Input: dimensioned drawing with shaded views. Units: mm. Origin: part minimum x, y, z. A direction names the side the tool comes from. Coordinates: 2 decimals unless noted, no trailing zeros. Order: outer loops, then holes, each group sorted by start corner. A loop starts at its lowest first (then second) coordinate and runs counter-clockwise, first axis right, second up. Notation, with made-up numbers: (81.5, 46.5) -> (106.5, 46.5) arc R13 cw to (106.5, 52.5) -> close; hole circle Ø9 at (-1.75, -29.5). An arc over 180 degrees is marked (long way). Write item = value, one per line. Start each with the question number.
Item 1: Set-up query: the marked faces 1, 2 and 3. Return all of +Z, -Z, +X, -X, +Y, -Y with unobstructed straight access to the full face (end or side cutting, diameter ignored); none if empty.
Item 2: Ray query, line 1 along Z through (x, y) = (68, 12); line 2 along X through (y, z) = (39.5, 4.75) (1 decimal); line 3 along Y through (x, z) = (29, 2.5) (1 decimal). Return the intervals inside material, ascending. Write a range as [from, to].
Item 3: Section query B-B (x = 36). Output: boundary loops of the cut face in (y, z), then the cut area to 3 significant figures.
Item 4: Section query A-A (y = 16.5). Output: boundary loops of the cut face in (x, z).
Item 5: Contact query for flat-ended pins moving along their axis: pin 1 (5 mm diameter, centred on x = 41, z = 6.5, fed in from -Y); pin 2 (4 mm diameter, centred on x = 9, z = 7.5, fed in from +Y); pin 3 (2 mm diameter, centred on x = 13.5, z = 1.5, fed in from +Y) (1 decimal); pin 4 (5 mm diameter, centred on x = 67.5, z = 7, fed in from +Y). Output: stop coordinate, or through.
Item 6: Section query D-D (y = 32). Output: boundary loops of the cut face in (x, z) (1 decimal), then the cut area to 3 significant figures.
Item 7: Section query C-C (z = 6.35). Output: boundary loops of the cut face in (x, y), then the cut area to 3 significant figures.
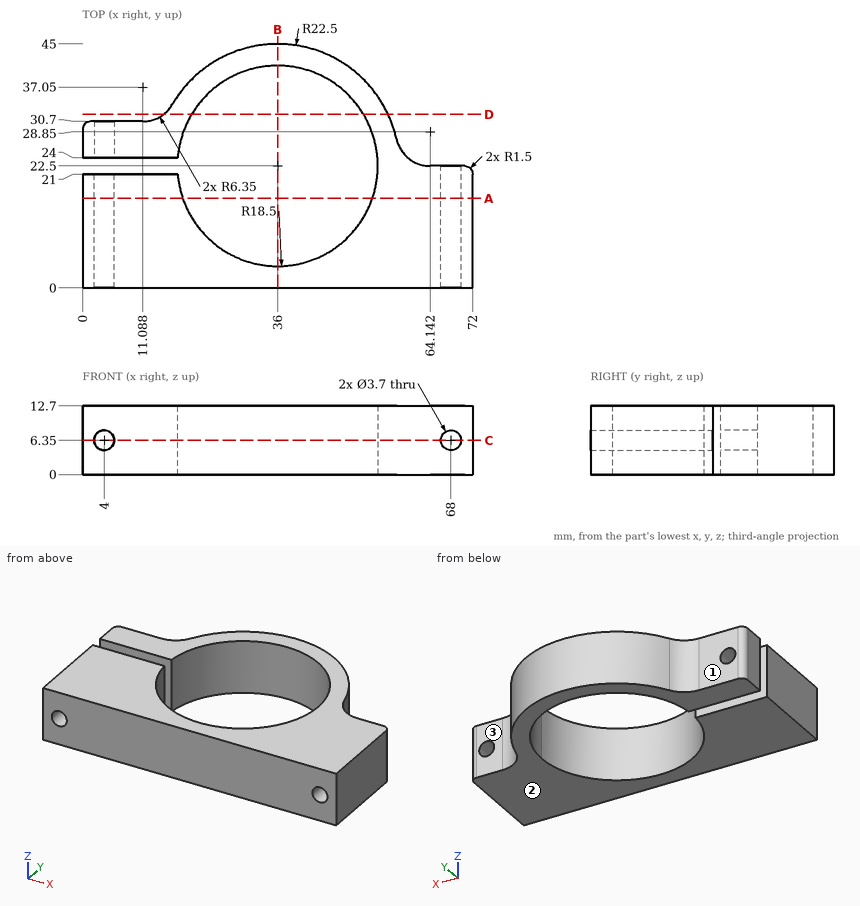
Computed:
q1.face_1 = +Z, -Z, -X, +Y
q1.face_2 = -Z, +X, -X, +Y, -Y
q1.face_3 = +Z, -Z, +X, +Y
q2.line_1 = [0, 4.5], [8.2, 12.7]
q2.line_2 = [21.3, 28.7], [43.3, 50.7]
q2.line_3 = [0, 5.4], [39.6, 43.9]
q3.outline = (0, 0) -> (4, 0) -> (4, 12.7) -> (0, 12.7) -> close; (41, 0) -> (45, 0) -> (45, 12.7) -> (41, 12.7) -> close
q3.area = 102 mm^2
q4.outline = (0, 0) -> (18.5, 0) -> (18.5, 12.7) -> (0, 12.7) -> close; (53.5, 0) -> (72, 0) -> (72, 12.7) -> (53.5, 12.7) -> close; hole circle Ø3.7 at (4, 6.35); hole circle Ø3.7 at (68, 6.35)
q5.pin_1 = 0
q5.pin_2 = 30.7
q5.pin_3 = 31.7
q5.pin_4 = 22.5
q6.outline = (14.9, 0) -> (20.1, 0) -> (20.1, 12.7) -> (14.9, 12.7) -> close; (51.9, 0) -> (56.4, 0) -> (56.4, 12.7) -> (51.9, 12.7) -> close
q6.area = 123 mm^2
q7.outline = (0, 0) -> (2.15, 0) -> (2.15, 21) -> (0, 21) -> close; (0, 24) -> (2.15, 24) -> (2.15, 30.7) -> (1.5, 30.7) arc R1.5 ccw to (0, 29.2) -> close; (5.85, 0) -> (66.15, 0) -> (66.15, 22.5) -> (64.14, 22.5) arc R6.35 cw to (57.95, 27.45) arc R22.5 ccw to (16.57, 33.85) arc R6.35 cw to (11.09, 30.7) -> (5.85, 30.7) -> (5.85, 24) -> (17.56, 24) arc R18.5 cw (long way) to (17.56, 21) -> (5.85, 21) -> close; (69.85, 0) -> (72, 0) -> (72, 21) arc R1.5 ccw to (70.5, 22.5) -> (69.85, 22.5) -> close
q7.area = 1,220 mm^2
